Design review of the part built by this model. Coordinates are the model's own, in mm. Face numbers are marked on the shaded views. A direction names the side the tool comes from. Round coordinates to 2 decimals unless told otherwise and drop trailing zeros. Loops run counter-clockwise (first coordinate to the right, second up) from the corner with the lowest first, then second, coordinate; pieces in that order, holes last. Notation, with made-up numbers: (11.25, 57) -> (61.25, 57) arc R12 ccw to (61.25, 65) -> close; hole circle Ø4 at (-39, 8). An arc over 180 degrees is marked (long way). Answer as CSV lines item,"result". Start each with the question number.
(1) For P1, Ø12, axis at y = 71.5, z = -24.5, coming from the +X side; P2, Ø12, axis at x = 7, y = 70.5, coming from the -Z side; P3, Ø24, axis at x = 30, y = 45, coming from the +Z side, all flat-tipped, find the tip position at first contact; note any pin that passes through.
(2) Take a section at A-A, the plane x = 30. Write out the cut boundary in (y, z).
(3) Take a section at C-C, the plane z = 22. Write out the cut boundary in (x, y).
(4) To check wall thickness, follow line 1 (Y direction, x = 57, z = -11); line 2 (Z direction, x = 30, y = 3.75); line 3 (Y direction, x = 30, z = 14.25). State the ranges of each line that lie inside material, in increasing order. Write a range as from..to.
(5) Take a section at D-D, the plane y = 28.5. Write out the cut boundary in (x, z), and give its area (3 significant figures).
(6) Machinability: for the marked faces 4, 5, 6, 7 and 8, which of the approach directions +Z, -Z, +X, -X, +Y, -Y give a long, thin tool a straight path to every point of the face, cutting with its end or side? Answer none if there is none.
(7) Draft analysis for pull direction Y (two halves, no side actions). For the marked faces 1, 2 and 3, state which applies: +Y half, -Y half, draft (parallel to the pull), parting line (faces both ways), or undercut.
(8) Take a section at B-B, the plane y = 62. Write out the cut boundary in (x, z), and give its area (3 significant figures).
from build123d import *

# Parameters (mm, degrees)
BOSS_EXTRUDE4_DEPTH     = 90
CUT_EXTRUDE1_DEPTH      = 69
CUT_EXTRUDE1_DEPTH_BACK = 18
SKETCH7_W               = 55.395667886
SKETCH7_H               = 70
SKETCH8_R               = 30
SKETCH8_R_2             = 20
BOSS_EXTRUDE5_DEPTH     = 30


with BuildPart() as part:
    # Sketch5 → Boss-Extrude4 (new body)
    with BuildSketch(Plane(origin=(0, 0, 0), x_dir=(1, 0, 0), z_dir=(0, 1, 0))):
        with BuildLine():
            Line((0, 30), (0, 0))
            Line((0, 0), (60, 0))
            Line((60, 0), (60, 30))
            Line((60, 30), (40, 30))
            ThreePointArc((40, 30), (30, 20), (20, 30))
            Line((20, 30), (0, 30))
        make_face()
        with BuildLine():
            ThreePointArc((60, 30), (30, 60), (0, 30))
            Line((0, 30), (20, 30))
            ThreePointArc((20, 30), (30, 40), (40, 30))
            Line((40, 30), (60, 30))
        make_face()
    extrude(amount=BOSS_EXTRUDE4_DEPTH)

    # Sketch7 → Cut-Extrude1 (cut, two sides: drawn at the far end of the back side and taken through both)
    with BuildSketch(Plane(origin=(0, 0, 0), x_dir=(0, 0, -1), z_dir=(1, 0, 0)).offset(-CUT_EXTRUDE1_DEPTH_BACK)):
        with Locations((37.697833943, 45)):
            Rectangle(SKETCH7_W, SKETCH7_H)
    extrude(amount=CUT_EXTRUDE1_DEPTH + CUT_EXTRUDE1_DEPTH_BACK, mode=Mode.SUBTRACT)

    # Sketch8 → Boss-Extrude5 (add)
    with BuildSketch(Plane.XY):
        with Locations((30, 45)):
            Circle(SKETCH8_R)
        with Locations((30, 45)):
            Circle(SKETCH8_R_2, mode=Mode.SUBTRACT)
    extrude(amount=BOSS_EXTRUDE5_DEPTH)


solid = part.part
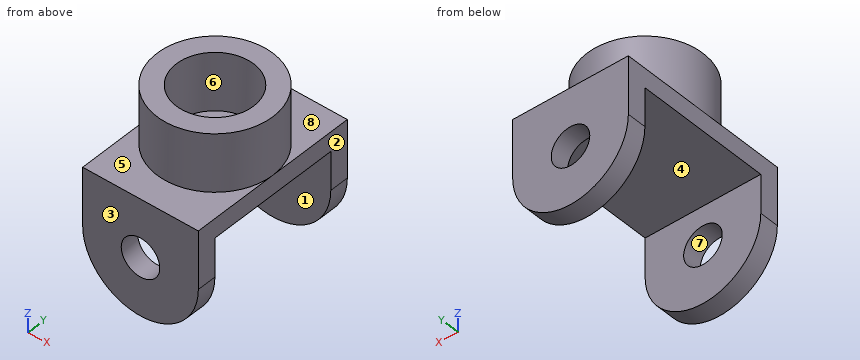
The answers:
1,P1,"through"
1,P2,"z = -10"
1,P3,"z = 0"
2,outline,"(0, -60) -> (10, -60) -> (10, -40) -> (0, -40) -> close; (0, -20) -> (10, -20) -> (10, -10) -> (80, -10) -> (80, -20) -> (90, -20) -> (90, 0) -> (75, 0) -> (75, 30) -> (65, 30) -> (65, 0) -> (25, 0) -> (25, 30) -> (15, 30) -> (15, 0) -> (0, 0) -> close; (80, -60) -> (90, -60) -> (90, -40) -> (80, -40) -> close"
3,outline,"circle Ø60 at (30, 45); hole circle Ø40 at (30, 45)"
4,line 1,"0..10, 80..90"
4,line 2,"-60..-40, -20..0"
4,line 3,"15..25, 65..75"
5,outline,"(0, -10) -> (60, -10) -> (60, 0) -> (55.05, 0) -> (55.05, 30) -> (41.3, 30) -> (41.3, 0) -> (18.7, 0) -> (18.7, 30) -> (4.95, 30) -> (4.95, 0) -> (0, 0) -> close"
5,area,"1,430 mm²"
6,face 4,"-Z, +X, -X"
6,face 5,"+Z, -Y"
6,face 6,"+Z"
6,face 7,"+Y, -Y"
6,face 8,"+Z, +Y"
7,face 1,"undercut"
7,face 2,"draft"
7,face 3,"-Y half"
8,outline,"(0, -10) -> (60, -10) -> (60, 0) -> (54.72, 0) -> (54.72, 30) -> (40.54, 30) -> (40.54, 0) -> (19.46, 0) -> (19.46, 30) -> (5.28, 30) -> (5.28, 0) -> (0, 0) -> close"
8,area,"1,450 mm²"
